Autodesk Fusion 360 part; units mm, degrees
sketch "Sketch1" plane through (0, 0, 0) normal (0, 0, 1) x (1, 0, 0)
  circle A0 centre (0, 0) radius 11
  circle A1 centre (0, 0) radius 12.5
  circle A2 centre (0, 0) radius 14.5
  line L0 (0, 0) -> (0, 14.5)
  line L1 (0, 0) -> (14.5, 0)
  line L2 (0, 0) -> (-14.5, 0)
  line L3 (0, 0) -> (0, -14.5)
  circle A3 centre (0, 14.5) radius 3.5
  circle A4 centre (14.5, 0) radius 3.5
  circle A5 centre (0, -14.5) radius 3.5
  circle A6 centre (-14.5, 0) radius 3.5
  circle A7 centre (-14.5, 0) radius 1.5
  circle A8 centre (0, 14.5) radius 1.5
  circle A9 centre (14.5, 0) radius 1.5
  circle A10 centre (0, -14.5) radius 1.5
  dimension "d1" = 22
  dimension "d2" = 25
  dimension "d3" = 29
  dimension "d4" = 7
  dimension "d5" = 3
  dimension "d6" = 3
  dimension "d7" = 3
  dimension "d8" = 3
extrude "Extrude1" add sketch "Sketch1" along normal blind 1 contours A0 A1 A4 A5 | A1 L1 A4 | A0 A1 A3 A4 | A1 L1 A4 | A1 L0 A3 | A0 A1 A3 A6 | A1 L0 A3 | A0 A1 A5 A6 | A1 L3 A5 | A1 L3 A5 | A1 A2 L1 A4 A9 | A1 A2 L1 A4 A9 | A1 A2 A3 A4 | A1 A2 A4 A5 | A1 L2 A6 | A1 L2 A6 | A1 A2 L0 A3 A8 | A1 A2 L0 A3 A8 | A1 A2 A3 A6 | A1 A2 L3 A5 A10 | A1 A2 L3 A5 A10 | A1 A2 A5 A6 | A2 A4 A9 | A1 A2 L2 A6 A7 | A1 A2 L2 A6 A7 | A2 A3 A8 | A2 A5 A10 | A2 A6 A7
sketch "Sketch2" plane through (0, 0, 1) normal (0, 0, 1) x (1, 0, 0)
  circle A0 centre (0, -14.5) radius 1.5
  circle A1 centre (14.5, 0) radius 1.5
  circle A2 centre (-14.5, 0) radius 1.5
  circle A3 centre (0, 14.5) radius 1.5
  circle A4 centre (0, 0) radius 11
  arc A5 (-3.4744, 14.0776) -> (-14.0776, 3.4744) centre (0, 0) ccw
  arc A6 (-14.0776, 3.4744) -> (-14.0776, -3.4744) centre (-14.5, 0) ccw
  arc A7 (-14.0776, -3.4744) -> (-3.4744, -14.0776) centre (0, 0) ccw
  arc A8 (-3.4744, -14.0776) -> (3.4744, -14.0776) centre (0, -14.5) ccw
  arc A9 (3.4744, -14.0776) -> (14.0776, -3.4744) centre (0, 0) ccw
  arc A10 (14.0776, -3.4744) -> (14.0776, 3.4744) centre (14.5, 0) ccw
  arc A11 (14.0776, 3.4744) -> (3.4744, 14.0776) centre (0, 0) ccw
  arc A12 (3.4744, 14.0776) -> (-3.4744, 14.0776) centre (0, 14.5) ccw
  circle A13 centre (0, 0) radius 11
  circle A14 centre (0, 0) radius 12.375
  circle A15 centre (0, 0) radius 14.5
  circle A16 centre (0, 14.5) radius 3.5
  circle A17 centre (14.5, 0) radius 3.5
  circle A18 centre (0, -14.5) radius 3.5
  circle A19 centre (-14.5, 0) radius 3.5
  dimension "d11" = 24.75
extrude "Extrude2" add sketch "Sketch2" along normal blind 1.25 contours A0 A8 A15 A18 | A0 A14 A15 A18 | A9 A14 A15 A17 A18 | A7 A14 A15 A18 A19 | A1 A10 A15 A17 | A1 A14 A15 A17 | A2 A6 A15 A19 | A2 A14 A15 A19 | A5 A14 A15 A16 A19 | A11 A14 A15 A16 A17 | A3 A12 A15 A16 | A3 A14 A15 A16
extrude "Extrude3" cut 1 faces at (-2.5265, -13.3305, 2.25) along direction (0, 0, -1) blind 1.25
sketch "Sketch3" plane through (0, 0, 1) normal (0, 0, 1) x (1, 0, 0)
  arc A0 (-3.4744, 14.0776) -> (-14.0776, 3.4744) centre (0, 0) ccw
  arc A1 (-14.0776, 3.4744) -> (-14.0776, -3.4744) centre (-14.5, 0) ccw
  arc A2 (-14.0776, -3.4744) -> (-3.4744, -14.0776) centre (0, 0) ccw
  arc A3 (-3.4744, -14.0776) -> (3.4744, -14.0776) centre (0, -14.5) ccw
  arc A4 (3.4744, -14.0776) -> (14.0776, -3.4744) centre (0, 0) ccw
  arc A5 (14.0776, -3.4744) -> (14.0776, 3.4744) centre (14.5, 0) ccw
  arc A6 (14.0776, 3.4744) -> (3.4744, 14.0776) centre (0, 0) ccw
  arc A7 (3.4744, 14.0776) -> (-3.4744, 14.0776) centre (0, 14.5) ccw
  circle A8 centre (0, 14.5) radius 1.5
  circle A9 centre (14.5, 0) radius 1.5
  circle A10 centre (-14.5, 0) radius 1.5
  circle A11 centre (0, -14.5) radius 1.5
  circle A12 centre (0, 0) radius 11
  circle A13 centre (0, 0) radius 3.05
  dimension "d16" = 6.1
extrude "Extrude4" add sketch "Sketch3" along normal blind 2 contours A0 A1 A2 A3 A4 A5 A6 A7 | A12
sketch "Sketch4" plane through (0, 0, 3) normal (0, 0, 1) x (1, 0, 0)
  circle A0 centre (-14.5, 0) radius 1.5
  circle A1 centre (0, 14.5) radius 1.5
  circle A2 centre (0, 0) radius 3.05
  circle A3 centre (0, -14.5) radius 1.5
  circle A4 centre (14.5, 0) radius 1.5
  arc A5 (3.4744, 14.0776) -> (-3.4744, 14.0776) centre (0, 14.5) ccw
  arc A6 (-3.4744, 14.0776) -> (-14.0776, 3.4744) centre (0, 0) ccw
  arc A7 (-14.0776, 3.4744) -> (-14.0776, -3.4744) centre (-14.5, 0) ccw
  arc A8 (-14.0776, -3.4744) -> (-3.4744, -14.0776) centre (0, 0) ccw
  arc A9 (-3.4744, -14.0776) -> (3.4744, -14.0776) centre (0, -14.5) ccw
  arc A10 (3.4744, -14.0776) -> (14.0776, -3.4744) centre (0, 0) ccw
  arc A11 (14.0776, -3.4744) -> (14.0776, 3.4744) centre (14.5, 0) ccw
  arc A12 (14.0776, 3.4744) -> (3.4744, 14.0776) centre (0, 0) ccw
  circle A13 centre (0, 0) radius 1.5
  dimension "d19" = 3
extrude "Extrude5" cut sketch "Sketch4" against normal blind 1 contours A5 A6 A7 A8 A9 A10 A11 A12
sketch "Sketch5" plane through (0, 0, 1) normal (0, 0, -1) x (-1, 0, 0)
  circle A0 centre (0, 0) radius 3.05
  circle A1 centre (0, 0) radius 11
  circle A2 centre (0, 0) radius 1.5
  dimension "d22" = 3
extrude "Extrude6" add sketch "Sketch5" against normal blind 1 contours A0
sketch "Sketch6" plane through (0, 0, 1) normal (0, 0, -1) x (-1, 0, 0)
  circle A0 centre (0, 0) radius 1.5
  circle A1 centre (0, 0) radius 11
  circle A2 centre (0, 0) radius 2.5
  dimension "d25" = 5
extrude "Extrude7" cut sketch "Sketch6" against normal blind 2 contours A2
sketch "Sketch7" plane through (0, 0, 1) normal (0, 0, -1) x (-1, 0, 0)
  circle A0 centre (0, 0) radius 2.5
  circle A1 centre (0, 0) radius 11
  circle A2 centre (0, 0) radius 5
  dimension "d28" = 10
extrude "Extrude8" cut sketch "Sketch7" against normal blind 4 contours A2
sketch "Sketch8" plane through (0, 0, 1) normal (0, 0, -1) x (-1, 0, 0)
  circle A0 centre (0, 0) radius 5
  circle A1 centre (0, 0) radius 11
  circle A2 centre (0, 0) radius 3.55
  dimension "d31" = 7.1
extrude "Extrude9" add sketch "Sketch8" against normal blind 1 contours A0
sketch "Sketch9" plane through (0, 0, 1) normal (0, 0, -1) x (-1, 0, 0)
  circle A0 centre (0, 0) radius 3.55
  circle A1 centre (0, 0) radius 11
  circle A2 centre (0, 0) radius 2.625
  dimension "d35" = 5.25
extrude "Extrude10" add sketch "Sketch9" along normal blind 1 contours A0 | A1
sketch "Sketch10" plane through (0, 0, 2) normal (0, 0, 1) x (1, 0, 0)
  circle A0 centre (0, 0) radius 3.55
  circle A1 centre (0, -14.5) radius 1.5
  circle A2 centre (14.5, 0) radius 1.5
  circle A3 centre (0, 14.5) radius 1.5
  circle A4 centre (-14.5, 0) radius 1.5
  arc A5 (14.0776, 3.4744) -> (3.4744, 14.0776) centre (0, 0) ccw
  arc A6 (3.4744, 14.0776) -> (-3.4744, 14.0776) centre (0, 14.5) ccw
  arc A7 (-3.4744, 14.0776) -> (-14.0776, 3.4744) centre (0, 0) ccw
  arc A8 (-14.0776, 3.4744) -> (-14.0776, -3.4744) centre (-14.5, 0) ccw
  arc A9 (-14.0776, -3.4744) -> (-3.4744, -14.0776) centre (0, 0) ccw
  arc A10 (-3.4744, -14.0776) -> (3.4744, -14.0776) centre (0, -14.5) ccw
  arc A11 (3.4744, -14.0776) -> (14.0776, -3.4744) centre (0, 0) ccw
  arc A12 (14.0776, -3.4744) -> (14.0776, 3.4744) centre (14.5, 0) ccw
  circle A13 centre (0, 0) radius 3.55
  circle A14 centre (0, 0) radius 4.5
  dimension "d38" = 9
extrude "Extrude11" add sketch "Sketch10" along normal blind 1 contours A14
chamfer "Chamfer1" distance 1 angle 45 1 edges at (-4.1955, 1.6273, 2)
sketch "Sketch11" plane through (0, 0, 3) normal (0, 0, 1) x (1, 0, 0)
  circle A0 centre (0, 0) radius 3.55
  circle A1 centre (0, 0) radius 4.5
  circle A2 centre (0, 0) radius 3.625
  dimension "d42" = 7.25
extrude "Extrude12" cut sketch "Sketch11" against normal blind 2 contours A2
extrude "Extrude13" add 1 faces at (4.1916, -0.2236, 3) along direction (0, 0, 1) blind 1
delete_face "DeleteFace1" 1 faces at (5.1409, -0.5144, 2.3333)
chamfer "Chamfer2" distance 2 angle 45 1 edges at (-4.1955, 1.6273, 2)
Could you check a few things on this model? Use its own coordinates, in mm. A direction names the side the tool comes from. Give positions to 0.01 mm unless a question says otherwise; leave off trailing zeros. Write each loop counter-clockwise with the first axis right and the second up, starting at its lowest first coordinate (ties: lowest second). Pieces come first, ordered by that corner, then holes. Notation, with made-up numbers: (3.5, -31) -> (26.5, -31) arc R15 cw to (26.5, -6) -> close; hole circle Ø4 at (29.25, 59.25). An arc over 180 degrees is marked (long way). Answer as a JSON object with one key per item and string values.
Q1. Which directions (+Z, -Z, +X, -X, +Y, -Y) give clear straight access to the entire face, cutting with the end or side of a thin tool? Please do faces 1 (the cylindrical face through (-2.5, -0.8, 0.5)), 2 (the cylindrical face through (1.7, 3.2, 2.5)).
Taken from the geometry:
{"face 1": "+Z, -Z", "face 2": "+Z"}
Q2. Will these pins go through, and if not, where does the flat tip stop? pin 1 Ø2.5 at (x, y) = (14.5, 0) entering from +Z; pin 2 Ø1 at (y, z) = (-3, 2) entering from -X; pin 3 Ø3.5 at (x, y) = (1.5, 1) entering from +Z; pin 4 Ø1 at (x, z) = (-1.5, 1.5) entering from +Y.
Taken from the geometry:
{"pin 1": "passes through", "pin 2": "stops at x = -16.95", "pin 3": "stops at z = 1", "pin 4": "stops at y = 17.85"}
Q3. We'd pull the mould along Y, two halves only. Please class faces 3 (the flat face through (-8, 0, 2)), 4 (the cylindrical face through (18, 0.1, 0.5)), 5 (the cylindrical face through (0, 16, 1)): released by +Y, released by -Y, zero draft, split by the parting line, or undercut.
Taken from the geometry:
{"face 3": "zero draft", "face 4": "split by the parting line", "face 5": "undercut"}
Q4. Suppose I cut it at A-A on x = 0. Count the separate pieces of the cut face and the enclosed holes in it, then the cut area to 3 significant figures.
Taken from the geometry:
{"separate pieces": "4", "enclosed holes": "0", "area": "55.0 mm²"}
Q5. Suppose I cut it at D-D on y = -10. Write out the boundary of the cut face in (x, z), then the cut area to 3 significant figures.
Taken from the geometry:
{"outline": "(-10.5, 0) -> (10.5, 0) -> (10.5, 2) -> (-10.5, 2) -> close", "area": "42.0 mm²"}
Q6. Please list where these lines run through material, in increasing order: L1, parallel to Y at x = 0, z = 1.25 (3 decimals); L2, parallel to Y at x = 0, z = 0.7 (3 decimals); L3, parallel to Y at x = 14.5, z = 1.55.
Taken from the geometry:
{"L1": "y = -18 to -16, -13 to -3.625, 3.625 to 13, 16 to 18", "L2": "y = -18 to -16, -13 to -2.625, 2.625 to 13, 16 to 18", "L3": "y = -3.5 to -1.5, 1.5 to 3.5"}
Q7. Suppose I cut it at B-B on y = -14.5. Write out the boundary of the cut face in (x, z), then the cut area to 3 significant figures.
Taken from the geometry:
{"outline": "(-3.5, 0) -> (-1.5, 0) -> (-1.5, 2) -> (-3.5, 2) -> close; (1.5, 0) -> (3.5, 0) -> (3.5, 2) -> (1.5, 2) -> close", "area": "8.00 mm²"}
